The model under review builds one solid part; all positions refer to its coordinate system, in mm. A direction names the side the tool comes from. Coordinates: 2 decimals unless noted, no trailing zeros. Write each loop counter-clockwise with the first axis right and the second up, starting at its lowest first coordinate (ties: lowest second). Pieces come first, ordered by that corner, then holes. Notation, with made-up numbers: (-38.75, 27) - (7.25, 27) arc R23 cw to (7.25, 35) - close; hole circle Ø10 at (-20.75, -12). An arc over 180 degrees is marked (long way). Answer as CSV lines item,"result". Start each with the question number.
Autodesk Inventor part; units mm, degrees
ref_plane "Work Plane1" through (0, 0, -37) normal (0, 0, 1) x (1, 0, 0)
ref_plane "Work Plane2" through (19.05, -19.05, 0) normal (-0.7071, -0.7071, 0) x (0, 0, -1)
ref_plane "YZ Plane" through (0, 0, 0) normal (1, 0, 0) x (0, 1, 0)
sketch "Sketch1" plane through (0, 0, 0) normal (0, 0, 1) x (1, 0, 0)
  line L0 (-19.05, 19.05) -> (19.05, 19.05)
  line L1 (19.05, 19.05) -> (19.05, -19.05)
  line L2 (19.05, -19.05) -> (-19.05, -19.05)
  line L3 (-19.05, -19.05) -> (-19.05, 19.05)
  point P0 (0, 0)
  dimension "d0" = 38.1
  dimension "d1" = 38.1
  dimension "d2" = 19.05
  dimension "d3" = 19.05
extrude "Extrusion1" add sketch "Sketch1" against normal blind 74
sketch "Sketch2" plane through (0, 0, 0) normal (0, 0, 1) x (1, 0, 0)
  line L0 (19.05, -19.05) -> (-19.05, -19.05)
  line L1 (19.05, 19.05) -> (19.05, -19.05)
  line L2 (-19.05, 19.05) -> (12.7, 19.05)
  line L3 (12.7, 19.05) -> (12.7, -12.7)
  line L4 (12.7, -12.7) -> (-19.05, -12.7)
  line L5 (-19.05, -12.7) -> (-19.05, 19.05)
  dimension "d6" = 6.35
  dimension "d7" = 6.35
extrude "Extrusion2" cut sketch "Sketch2" against normal through all
ref_plane "Work Plane1" through (0, 0, -37) normal (0, 0, 1) x (1, 0, 0)
fillet "Fillet1" radius 3.81 3 edges at (12.7, 19.05, -37) (-19.05, -12.7, -37) (12.7, -12.7, -37)
ref_plane "Work Plane2" through (19.05, -19.05, 0) normal (-0.7071, -0.7071, 0) x (0, 0, -1)
sketch "Sketch7" plane through (12.7, -8.89, 0) normal (-1, 0, 0) x (0, 0, 1)
  line L0 (0, -10.16) -> (-74, -10.16)
  line L1 (0, -10.16) -> (-74, -10.16)
  line L2 (-37, 35.56) -> (-37, -17.78)
  point P0 (-17, 9.84)
  point P1 (-17.95, 8.89)
  dimension "d29" = 20
  dimension "d30" = 19.05
  dimension "d31" = 20
  dimension "d32" = 19.05
hole "Hole2" at (12.7, 0.95, -17) at (12.7, 0, -17.95) direction (1, 0, 0) diameter 8.4 end through all
mirror "Mirror4" about plane through (0, 0, -37) normal (0, 0, 1) of "Hole2"
mirror "Mirror5" about plane through (19.05, -19.05, 0) normal (-0.7071, -0.7071, 0) of "Hole2", "Mirror4"
sketch "Sketch9" plane through (12.7, -8.89, 0) normal (-1, 0, 0) x (0, 0, 1)
  arc A0 (-20.4066, 12.2966) -> (-14.5434, 6.4334) centre (-17.95, 8.89) ccw
  arc A1 (-14.5434, 6.4334) -> (-20.4066, 12.2966) centre (-17, 9.84) ccw
  line L0 (-19.9698, 12.8098) -> (-20.9198, 11.8598)
  line L1 (-14.9802, 5.9202) -> (-14.0302, 6.8702)
extrude "Extrusion7" cut sketch "Sketch9" against normal through all contours A0 L0 A1 | A0 A1 L1
mirror "Mirror6" about plane through (0, 0, -37) normal (0, 0, 1) of "Extrusion7"
mirror "Mirror7" about plane through (19.05, -19.05, 0) normal (-0.7071, -0.7071, 0) of "Extrusion7", "Mirror6"
equation "\"d1\" = d0"
equation "\"d7\" = d6"
properties part number "28-604" material "Aluminum-6061"
(1) Add section C-C on y = 0.95. Give the boundary of the cut face in (x, z), then the cut area to 3 significant figures.
(2) Wall thickness on line 1 (Z direction, x = 15, y = 4.5); line 2 (X direction, y = 4.5, z = -4.5); line 3 (Z direction, x = 2, y = -16): over which ranges is each line inside the solid? List them lowest first.
(3) Add section A-A on z = -17. Give the boundary of the cut face in (x, y), then the cut area to 3 significant figures.
(4) Add section B-B on x = 0. Give the boundary of the cut face in (y, z).
(5) For pin 1 (12 mm diameter, centred on x = -8, z = -30.5, fed in from +Y); pin 2 (19.5 mm diameter, centred on y = 5, z = -50, fed in from -X); pin 3 (6 mm diameter, centred on y = -12.5, z = -62.5, fed in from -X), all flat-tipped, find the tip position at first contact; note any pin that passes through.
(6) The part is to be moulded in two halves that separate along Y. For faces 1 (the cylindrical face through (15.919, -3.034, -20.854)), 2 (the flat face through (18, 19.05, -36)), 3 (the flat face through (19.05, 0, -36)), say which applies: released by +Y, released by -Y, zero draft, split by the parting line, or undercut.
(7) Add section D-D on z = -38. Give the boundary of the cut face in (x, y).
(8) For faces 4 (the cylindrical face through (-3.854, -15.919, -13.966)), 5 (the flat face through (-3, -12.7, -36)), list the 3-axis set-ups (+Z, -Z, +X, -X, +Y, -Y) from which the entire face can be reached by the end or side of a thin tool; tool diameter is ignored.
Reported:
1,outline,"(12.7, -74) - (19.05, -74) - (19.05, -61.2) - (12.7, -61.2) - close; (12.7, -51.96) - (19.05, -51.96) - (19.05, -22.04) - (12.7, -22.04) - close; (12.7, -12.8) - (19.05, -12.8) - (19.05, 0) - (12.7, 0) - close"
1,area,"353 mm²"
2,line 1,"-74 to -59.24, -54.76 to -19.24, -14.76 to 0"
2,line 2,"12.7 to 19.05"
2,line 3,"-74 to -59.99, -52.36 to -21.64, -14.01 to 0"
3,outline,"(-19.05, -19.05) - (-5.15, -19.05) - (-5.15, -12.7) - (-15.24, -12.7) arc R3.81 ccw to (-19.05, -16.51) - close; (4.09, -19.05) - (19.05, -19.05) - (19.05, -4.09) - (12.7, -4.09) - (12.7, -8.89) arc R3.81 cw to (8.89, -12.7) - (4.09, -12.7) - close; (12.7, 5.15) - (19.05, 5.15) - (19.05, 19.05) - (16.51, 19.05) arc R3.81 ccw to (12.7, 15.24) - close"
3,area,"323 mm²"
4,outline,"(-19.05, -74) - (-12.7, -74) - (-12.7, -61.09) - (-19.05, -61.09) - close; (-19.05, -51.85) - (-12.7, -51.85) - (-12.7, -22.15) - (-19.05, -22.15) - close; (-19.05, -12.91) - (-12.7, -12.91) - (-12.7, 0) - (-19.05, 0) - close"
5,pin 1,"y = -12.7"
5,pin 2,"x = 12.7"
5,pin 3,"x = -18.91"
6,face 1,"undercut"
6,face 2,"released by +Y"
6,face 3,"zero draft"
7,outline,"(-19.05, -19.05) - (19.05, -19.05) - (19.05, 19.05) - (16.51, 19.05) arc R3.81 ccw to (12.7, 15.24) - (12.7, -8.89) arc R3.81 cw to (8.89, -12.7) - (-15.24, -12.7) arc R3.81 ccw to (-19.05, -16.51) - close"
8,face 4,"+Y, -Y"
8,face 5,"+Z, -Z, -X, +Y"
